For this review, use the dimensioned drawing (mm, ordinates from the lowest corner) and the shaded views. Round coordinates to 2 decimals unless told otherwise and drop trailing zeros. Write each loop counter-clockwise with the first axis right and the second up, starting at its lowest first coordinate (ties: lowest second). Pieces come first, ordered by that corner, then holes. Notation, with made-up numbers: (58, 84.5) -> (113, 84.5) arc R16 cw to (113, 103.5) -> close; hole circle Ø3 at (69, -9.75). An arc over 180 degrees is marked (long way). Answer in a Markdown table with one row per item. Add a question column.
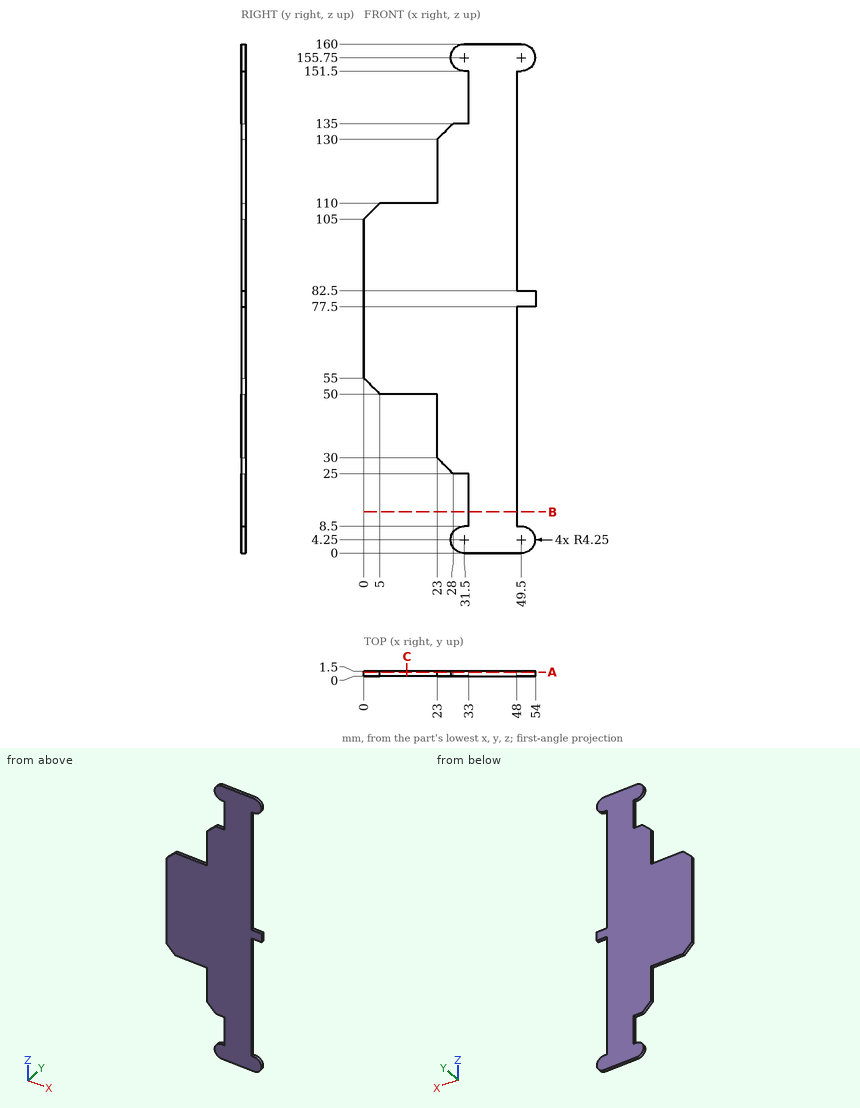
1. We need section B-B (z = 13). Write out the cut boundary in (x, y).
2. For L1, parallel to Z at x = 32.5, y = 0.25; L2, parallel to Z at x = 50.5, y = 1.15; L3, parallel to X at y = 0.4, z = 137.5, list the stretches that pass through material, from the lowest coordinate up. Write a range as [from, to].
3. We need section A-A (y = 1.2). Write out the cut boundary in (x, z), plus the area to 3 significant figures.
4. We need section C-C (x = 13.5). Write out the cut boundary in (y, z), plus the area to 3 significant figures.
5. Clearance check with a flat-ended pin moving along its axis: pin 1 Ø0.8 at (x, y) = (30, 0.5) entering from +Z. State where the tip first meets the part, or that it passes through.
Response:
| question | item | result |
|---|---|---|
| 1 | outline | (33, 0) -> (48, 0) -> (48, 1.5) -> (33, 1.5) -> close |
| 2 | L1 | [0, 8.5], [25, 135], [151.5, 160] |
| 2 | L2 | [0.12, 8.38], [77.5, 82.5], [151.62, 159.88] |
| 2 | L3 | [33, 48] |
| 3 | outline | (0, 55) -> (5, 50) -> (23, 50) -> (23, 30) -> (28, 25) -> (33, 25) -> (33, 8.5) -> (31.5, 8.5) arc R4.25 ccw to (31.5, 0) -> (49.5, 0) arc R4.25 ccw to (49.5, 8.5) -> (48, 8.5) -> (48, 77.5) -> (54, 77.5) -> (54, 82.5) -> (48, 82.5) -> (48, 151.5) -> (49.5, 151.5) arc R4.25 ccw to (49.5, 160) -> (31.5, 160) arc R4.25 ccw to (31.5, 151.5) -> (33, 151.5) -> (33, 135) -> (28, 135) -> (23, 130) -> (23, 110) -> (5, 110) -> (0, 105) -> close |
| 3 | area | 5,020 mm2 |
| 4 | outline | (0, 50) -> (1.5, 50) -> (1.5, 110) -> (0, 110) -> close |
| 4 | area | 90.0 mm2 |
| 5 | pin 1 | z = 159.86 |
